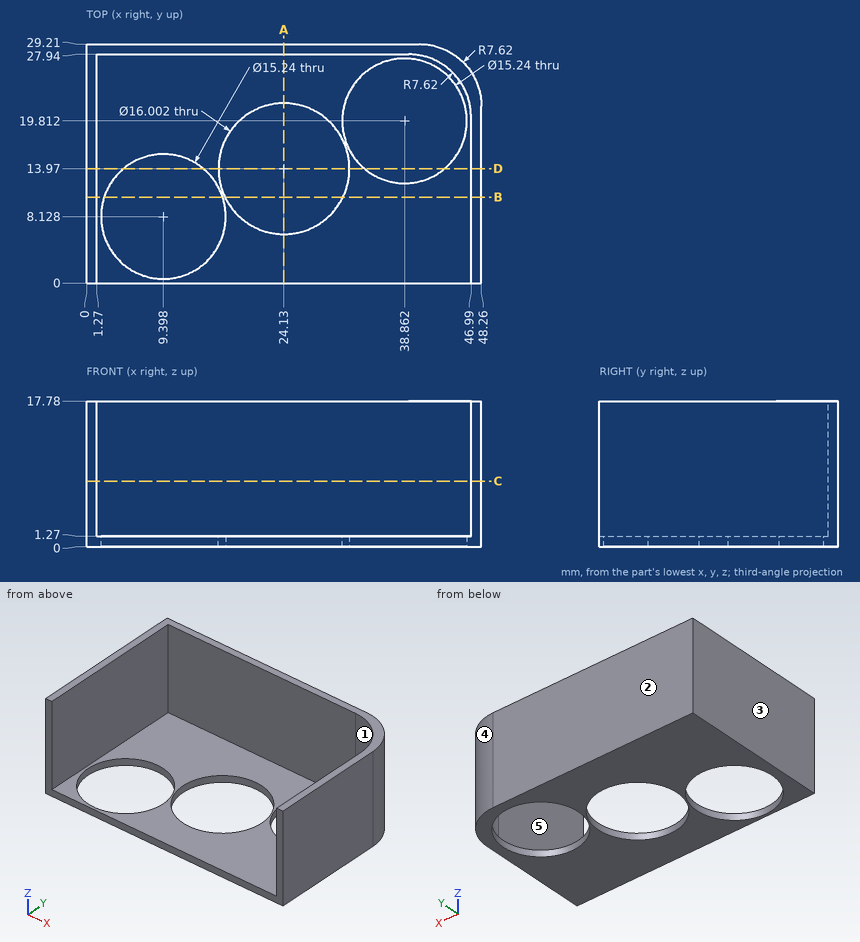
The drawing under review shows one solid part. Ordinate dimensions are in mm from its lowest x, y, z. A direction names the side the tool comes from. Coordinates: 2 decimals unless noted, no trailing zeros. Loops run counter-clockwise (first coordinate to the right, second up) from the corner with the lowest first, then second, coordinate; pieces in that order, holes last. Notation, with made-up numbers: (-33.75, 66.25) - (1.25, 66.25) arc R27 cw to (1.25, 97.25) - close; hole circle Ø8 at (-26, -2.5). An arc over 180 degrees is marked (long way). Return JSON: item names as keys, results as strings.
Item 1: For the marked faces 1 and 2, list the 3-axis set-ups (+Z, -Z, +X, -X, +Y, -Y) from which the entire face can be reached by the end or side of a thin tool; tool diameter is ignored.
Determined:
{"face 1": "+Z, -Y", "face 2": "+Z, -Z, +X, -X, +Y"}
Item 2: Take a section at A-A (x = 24.13). Give the boundary of the cut face in (y, z).
Determined:
{"outline": "(0, 0) - (5.97, 0) - (5.97, 1.27) - (0, 1.27) - close; (21.97, 0) - (29.21, 0) - (29.21, 17.78) - (27.94, 17.78) - (27.94, 1.27) - (21.97, 1.27) - close"}
Item 3: Insertion check: pin 1 (8.5 mm diameter, centred on x = 20.5, z = 6.5, fed in from -Y); pin 2 (8.5 mm diameter, centred on x = 34, y = 18.5, fed in from +Z); pin 3 (12 mm diameter, centred on x = 9.398, y = 8.128, fed in from -Z). Each pin has a flat end and moves straight along its axis. Give the tip position at first contact, or say it passes through.
Determined:
{"pin 1": "stops at y = 27.94", "pin 2": "stops at z = 1.27", "pin 3": "passes through"}
Item 4: Take a section at D-D (y = 13.97). Give the boundary of the cut face in (x, z), then the cut area to 3 significant figures.
Determined:
{"outline": "(0, 0) - (4.51, 0) - (4.51, 1.27) - (1.27, 1.27) - (1.27, 17.78) - (0, 17.78) - close; (14.29, 0) - (16.13, 0) - (16.13, 1.27) - (14.29, 1.27) - close; (32.13, 0) - (33.97, 0) - (33.97, 1.27) - (32.13, 1.27) - close; (43.75, 0) - (48.26, 0) - (48.26, 17.78) - (46.99, 17.78) - (46.99, 1.27) - (43.75, 1.27) - close", "area": "58.0 mm2"}
Item 5: Take a section at B-B (y = 10.5). Give the boundary of the cut face in (x, z), then the cut area to 3 significant figures.
Determined:
{"outline": "(0, 0) - (2.16, 0) - (2.16, 1.27) - (1.27, 1.27) - (1.27, 17.78) - (0, 17.78) - close; (16.64, 0) - (16.92, 0) - (16.92, 1.27) - (16.64, 1.27) - close; (31.34, 0) - (48.26, 0) - (48.26, 17.78) - (46.99, 17.78) - (46.99, 1.27) - (31.34, 1.27) - close", "area": "66.5 mm2"}
Item 6: Take a section at C-C (z = 8). Give the boundary of the cut face in (x, y), then the cut area to 3 significant figures.
Determined:
{"outline": "(0, 0) - (1.27, 0) - (1.27, 27.94) - (39.37, 27.94) arc R7.62 cw to (46.99, 20.32) - (46.99, 0) - (48.26, 0) - (48.26, 21.59) arc R7.62 ccw to (40.64, 29.21) - (0, 29.21) - close", "area": "132 mm2"}
Item 7: Mouldability with a two-part tool opening along X and no side actions: class the marked faces 3, 4 and 5 as pulls with the +X half, pulls with the -X half, needs draft (parallel to the pull), parting line crosses it, or undercut.
Determined:
{"face 3": "pulls with the -X half", "face 4": "pulls with the +X half", "face 5": "undercut"}
Item 8: For line 1 (X direction, y = 15.25, z = 6); line 2 (Y direction, x = 24.13, z = 0.4); line 3 (Y direction, x = 20.5, z = 6.5), list the stretches that pass through material, from the lowest coordinate up.
Determined:
{"line 1": "x = 0 to 1.27, 46.99 to 48.26", "line 2": "y = 0 to 5.97, 21.97 to 29.21", "line 3": "y = 27.94 to 29.21"}
